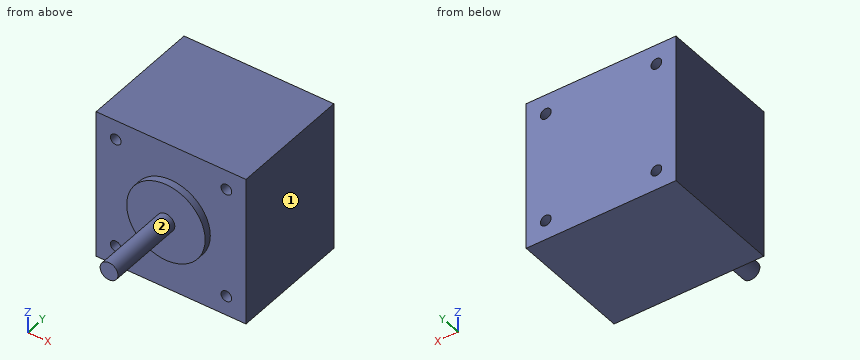
from build123d import *

# Parameters (mm, degrees)
F0_W     = 42
F0_H     = 42
F0_R     = 1.5
F0_R_2   = 11
F0_R_3   = 2.5
F1_DEPTH = 34
F2_DEPTH = 24
F3_DEPTH = 2


with BuildPart() as f1:
    # F0 (on Front) → F1 (new body)
    with BuildSketch(Plane.XZ):
        with Locations((-21, 21)):
            Rectangle(F0_W, F0_H)
        with Locations((-36.5, 5.5)):
            Circle(F0_R, mode=Mode.SUBTRACT)
        with Locations((-5.5, 5.5)):
            Circle(F0_R, mode=Mode.SUBTRACT)
        with Locations((-36.5, 36.5)):
            Circle(F0_R, mode=Mode.SUBTRACT)
        with Locations((-21, 21)):
            Circle(F0_R_2, mode=Mode.SUBTRACT)
        with Locations((-5.5, 36.5)):
            Circle(F0_R, mode=Mode.SUBTRACT)
        with Locations((-21, 21)):
            Circle(F0_R_2)
        with Locations((-21, 21)):
            Circle(F0_R_3, mode=Mode.SUBTRACT)
        with Locations((-21, 21)):
            Circle(F0_R_3)
    extrude(amount=-F1_DEPTH)

    # F0 (on Front) → F2 (join)
    with BuildSketch(Plane.XZ):
        with Locations((-21, 21)):
            Circle(F0_R_3)
    extrude(amount=F2_DEPTH)

    # F0 (on Front) → F3 (join)
    with BuildSketch(Plane.XZ):
        with Locations((-21, 21)):
            Circle(F0_R_2)
        with Locations((-21, 21)):
            Circle(F0_R_3, mode=Mode.SUBTRACT)
    extrude(amount=F3_DEPTH)


solid = f1.part
Source: CAD feature listing. Evaluate the final solid. Frame: model axes, mm. Face numbers are marked on the shaded views. A direction names the side the tool comes from. Coordinates: 2 decimals unless noted, no trailing zeros. Order: outer loops, then holes, each group sorted by start corner. A loop starts at its lowest first (then second) coordinate and runs counter-clockwise, first axis right, second up. Notation, with made-up numbers: M -38.5,35 L -1.5,35 A23 ccw -1.5,61 Z; hole C 49.25,-14 d10. An arc over 180 degrees is marked long. Write each question's results on one line, items separated by ' | '. Start each with the question number.
Item 1: First-contact query: pin 1 Ø1.5 at (x, z) = (-12.5, 23.5) entering from -Y; pin 2 Ø6 at (y, z) = (-16, 27.5) entering from -X. Flat tips, straight axial feed; report the tip coordinate or a pass-through.
Item 2: Line query: probe 1 along Z at (x, y) = (-36.5, 8); probe 2 along X at (y, z) = (13, 36); probe 3 along Y at (x, z) = (-19.5, 28). Output: solid intervals per line, ascending.
Item 3: Cut plane B-B (x = -5.5). Return loops of the section in (y, z).
Item 4: Cut plane D-D (x = -21). Return loops of the section in (y, z).
Item 5: Cut plane C-C (y = 20). Return loops of the section in (x, z).
Item 6: Cut plane A-A (z = 36.5). Return loops of the section in (x, y).
Item 7: Set-up query: the marked faces 1 and 2. Return all of +Z, -Z, +X, -X, +Y, -Y with unobstructed straight access to the full face (end or side cutting, diameter ignored); none if empty.
Checked values:
1) pin 1: stops at y = -2 | pin 2: passes through
2) probe 1: z = 0 to 4, 7 to 35, 38 to 42 | probe 2: x = -42 to -37.91, -35.09 to -6.91, -4.09 to 0 | probe 3: y = -2 to 34
3) outline: M 0,0 L 34,0 L 34,4 L 0,4 Z; M 0,7 L 34,7 L 34,35 L 0,35 Z; M 0,38 L 34,38 L 34,42 L 0,42 Z
4) outline: M -24,18.5 L -2,18.5 L -2,10 L 0,10 L 0,0 L 34,0 L 34,42 L 0,42 L 0,32 L -2,32 L -2,23.5 L -24,23.5 Z
5) outline: M -42,0 L 0,0 L 0,42 L -42,42 Z; hole C -36.5,5.5 d3; hole C -36.5,36.5 d3; hole C -5.5,5.5 d3; hole C -5.5,36.5 d3
6) outline: M -42,0 L -38,0 L -38,34 L -42,34 Z; M -35,0 L -7,0 L -7,34 L -35,34 Z; M -4,0 L 0,0 L 0,34 L -4,34 Z
7) face 1: +Z, -Z, +X, +Y, -Y | face 2: -Y
